Geometry check sheet. Reference: the model listing, model coordinates, mm. Coordinates: 2 decimals unless noted, no trailing zeros. Order: outer loops, then holes, each group sorted by start corner. A loop starts at its lowest first (then second) coordinate and runs counter-clockwise, first axis right, second up. Notation, with made-up numbers: (57, 2) - (68, 2) arc R23 ccw to (68, 22) - close; hole circle Ø8 at (15.25, -28.5). An arc over 180 degrees is marked (long way). One line per item, written item: value. Start each with the question number.
Autodesk Inventor part; units mm, degrees
sketch "Sketch1" plane through (0, 0, 0) normal (0, 0, 1) x (1, 0, 0)
  line L0 (1.8764, 3.25) -> (3.7528, 0)
  line L1 (3.7528, 0) -> (1.8764, -3.25)
  line L2 (1.8764, -3.25) -> (-1.8764, -3.25)
  line L3 (-1.8764, -3.25) -> (-3.7528, 0)
  line L4 (-3.7528, 0) -> (-1.8764, 3.25)
  line L5 (-1.8764, 3.25) -> (1.8764, 3.25)
  point P0 (0, 0)
  point P1 (0, 0)
  dimension "d0" = 6.5
extrude "Extrusion1" add sketch "Sketch1" along normal blind 4.5
properties part number "servo_metal_600TVL_shaft_nut"
Q1. Cross-section at C-C, the plane x = 2.5. Enter the section's corners in (y, z), and give its area (3 significant figures).
Q2. Cross-section at A-A, the plane z = 1.9. Enter the section's corners in (x, y), and give its area (3 significant figures).
Q3. Material ranges on probe 1 along X at (y, z) = (2.25, 4); probe 2 along X at (y, z) = (2, 3); probe 3 along Y at (x, z) = (-2, 1.7), recorded low to high.
Q4. Cross-section at B-B, the plane y = -0.25. Enter the section's corners in (x, z), and give its area (3 significant figures).
Q5. Gauge pin test, flat end, axial feed: P1, Ø1.5, axis at x = -2.5, z = 3.5, coming from the +Y side. Record the tip position at first contact, or that the pin passes through.
Check result:
1. outline: (-2.17, 0) - (2.17, 0) - (2.17, 4.5) - (-2.17, 4.5) - close
1. area: 19.5 mm2
2. outline: (-3.75, 0) - (-1.88, -3.25) - (1.88, -3.25) - (3.75, 0) - (1.88, 3.25) - (-1.88, 3.25) - close
2. area: 36.6 mm2
3. probe 1: x = -2.45 to 2.45
3. probe 2: x = -2.6 to 2.6
3. probe 3: y = -3.04 to 3.04
4. outline: (-3.61, 0) - (3.61, 0) - (3.61, 4.5) - (-3.61, 4.5) - close
4. area: 32.5 mm2
5. P1: stops at y = 3.25
